The model under review builds one solid part; all positions refer to its coordinate system, in mm. A direction names the side the tool comes from. Coordinates: 2 decimals unless noted, no trailing zeros. Order: outer loops, then holes, each group sorted by start corner. A loop starts at its lowest first (then second) coordinate and runs counter-clockwise, first axis right, second up. Notation, with made-up numbers: (88, 68) - (109, 68) arc R22 ccw to (109, 91) - close; hole circle Ø7 at (18, 53). An arc over 180 degrees is marked (long way). Answer in a Markdown table with one row per item.
Autodesk Inventor part; units mm, degrees
ref_plane "YZ Plane" through (0, 0, 0) normal (1, 0, 0) x (0, 1, 0)
ref_plane "XZ Plane" through (0, 0, 0) normal (0, 1, 0) x (-1, 0, 0)
ref_plane "XY Plane" through (0, 0, 0) normal (0, 0, 1) x (1, 0, 0)
sketch "Sketch1" plane through (0, 0, 0) normal (0, 1, 0) x (-1, 0, 0)
  line L0 (-41.5, -207.85) -> (-41.5, -204.85)
  line L1 (-44.5, -201.85) -> (-51.2, -201.85)
  line L2 (-54.2, -204.85) -> (-54.2, -207.85)
  line L3 (-57.2, -210.85) -> (-61.5, -210.85)
  arc A0 (-41.5, -207.85) -> (-38.5, -210.85) centre (-38.5, -207.85) ccw
  arc A1 (-41.5, -204.85) -> (-44.5, -201.85) centre (-44.5, -204.85) ccw
  arc A2 (-51.2, -201.85) -> (-54.2, -204.85) centre (-51.2, -204.85) ccw
  arc A3 (-57.2, -210.85) -> (-54.2, -207.85) centre (-57.2, -207.85) ccw
  line L4 (41.5, -207.85) -> (41.5, -204.85)
  line L5 (44.5, -201.85) -> (51.2, -201.85)
  line L6 (54.2, -204.85) -> (54.2, -207.85)
  line L7 (61.5, -210.85) -> (57.2, -210.85)
  line L8 (38.5, -210.85) -> (-38.5, -210.85)
  arc A4 (54.2, -207.85) -> (57.2, -210.85) centre (57.2, -207.85) ccw
  arc A5 (54.2, -204.85) -> (51.2, -201.85) centre (51.2, -204.85) ccw
  arc A6 (44.5, -201.85) -> (41.5, -204.85) centre (44.5, -204.85) ccw
  arc A7 (38.5, -210.85) -> (41.5, -207.85) centre (38.5, -207.85) ccw
  line L9 (44.75, 48.15) -> (25.05, 48.15)
  line L10 (25.05, 48.15) -> (25.05, 57.15)
  line L11 (25.05, 57.15) -> (44.75, 57.15)
  line L12 (44.75, 57.15) -> (44.75, 48.15)
  line L13 (-25.05, 48.15) -> (-44.75, 48.15)
  line L14 (-44.75, 48.15) -> (-44.75, 57.15)
  line L15 (-44.75, 57.15) -> (-25.05, 57.15)
  line L16 (-25.05, 57.15) -> (-25.05, 48.15)
  line L17 (44.75, 48.15) -> (63, 48.15)
  line L18 (25.05, 48.15) -> (-25.05, 48.15)
  line L19 (-44.75, 48.15) -> (-63, 48.15)
  line L20 (63, -209.35) -> (63, 48.15)
  line L21 (-63, -209.35) -> (-63, 48.15)
  arc A8 (61.5, -210.85) -> (63, -209.35) centre (61.5, -209.35) ccw
  arc A9 (-63, -209.35) -> (-61.5, -210.85) centre (-61.5, -209.35) ccw
  point P0 (0, 0)
  point P1 (-47.85, -207.15)
  point P2 (47.85, -207.85)
  point P3 (34.9, 57.15)
  point P4 (-34.9, 57.15)
  point P5 (-59.35, -210.85)
  point P6 (0, -210.85)
  point P7 (59.35, -210.85)
  point P8 (0, 48.15)
  point P9 (-47.85, -201.85)
  point P10 (47.85, -201.85)
  dimension "d3" = 12.7
  dimension "d5" = 3
  dimension "d7" = 12.7
  dimension "d9" = 3
  dimension "d10" = 9
  dimension "d11" = 19.7
  dimension "d13" = 9
  dimension "d14" = 19.7
  dimension "d16" = 1.5
  dimension "d17" = 126
  dimension "d20" = 18.25
  dimension "d21" = 18.25
  dimension "d22" = 57.15
  dimension "d23" = 9
  dimension "d24" = 9
  dimension "d27" = 250
  dimension "d28" = 250
  dimension "d53" = 83
  dimension "d54" = 3.7
extrude "base" add sketch "Sketch1" along normal blind 5
sketch "Sketch2" plane through (0, 5, 0) normal (0, 1, 0) x (1, 0, 0)
  circle A0 centre (0, -26.65) radius 9
  line L0 (-25.05, -48.15) -> (25.05, -48.15)
  line L1 (0, -26.65) -> (-33, -26.65) construction
  point P0 (0, 0)
  dimension "d31" = 18
  dimension "d32" = 21.5
  dimension "d52" = 33
extrude "Poke Hole" cut sketch "Sketch2" against normal up to surface (5 mm away)
pattern_linear "Rectangular Pattern1" count 2 spacing 33 along (0, 0, -1) of "Poke Hole"
sketch "Sketch3" plane through (0, 5, 0) normal (0, 1, 0) x (1, 0, 0)
  circle A0 centre (0, 17.45) radius 1.5
  circle A1 centre (0, 6.35) radius 9
  circle A2 centre (-9.6129, 0.8) radius 1.5
  circle A3 centre (9.6129, 0.8) radius 1.5
  point P0 (0, 0)
  point P1 (0, 6.35)
  dimension "d41" = 3
  dimension "d42" = 11.1
  dimension "d45" = 360
extrude "Mount Holes" cut sketch "Sketch3" against normal up to surface (5 mm away) contours A0 | A2 | A3
pattern_linear "Rectangular Pattern2" count 2 spacing 33 along (0, 0, 1) of "Mount Holes"
sketch "Sketch4" plane through (0, 5, 0) normal (0, 1, 0) x (1, 0, 0)
  circle A0 centre (-44.775, -21.6952) radius 1.65
  circle A1 centre (-25.025, -21.6952) radius 1.65
  line L0 (-44.775, -21.6952) -> (-25.025, -21.6952) construction
  circle A2 centre (0, 17.45) radius 1.5 construction
  circle A3 centre (-34.9, 21.6952) radius 1.65
  line L1 (-63, 209.35) -> (-63, -48.15)
  line L2 (-25.05, -48.15) -> (25.05, -48.15) construction
  line L3 (-44.75, -48.15) -> (-25.05, -48.15) construction
  line L4 (-44.775, -21.6952) -> (-25.025, -21.6952) construction
  line L5 (-34.9, 21.6952) -> (-34.9, -21.6952) construction
  point P0 (0, 0)
  point P1 (-34.9, -48.15)
  point P2 (-34.9, 0)
  dimension "d55" = 3.3
  dimension "d56" = 3.3
  dimension "d57" = 19.75
  dimension "d58" = 3.3
  dimension "d59" = 44.5
extrude "PCB mount holes" cut sketch "Sketch4" against normal up to surface (5 mm away)
pattern_linear "Rectangular Pattern3" count 2 spacing 66 along (1, 0, 0) of "PCB mount holes"
equation "\"d7\" = d3"
equation "\"d9\" = d5"
equation "\"d10\" = d23"
equation "\"d13\" = d23"
equation "\"d14\" = d11"
equation "\"d21\" = d20"
equation "\"d24\" = d23"
equation "\"d37\" = d52"
equation "\"d40\" = d52"
equation "\"d51\" = d52"
equation "\"d56\" = d55"
equation "\"d58\" = d55"
equation "\"d66\" = 2 * d52"
properties part number "front_wall_2poke" material "PPS Plastic"
Item 1: Mouldability with a two-part tool opening along X and no side actions: class faces 6 (the face through (-63, 2, -82)), 7 (the face through (54, 2, 48.15)), 8 (the face through (-25.05, 2, 53)), 9 (the face through (63, 2, -82)) as +X half, -X half, draft (parallel to the pull), parting line (faces both ways), or undercut.
Check values:
| item | result |
|---|---|
| face 6 | -X half |
| face 7 | draft |
| face 8 | undercut |
| face 9 | +X half |
Item 2: We need section A-A, the plane x = -18. Write out the cut boundary in (y, z), then the cut area to 4 significant figures.
Check values:
| item | result |
|---|---|
| outline | (0, -210.85) - (5, -210.85) - (5, 48.15) - (0, 48.15) - close |
| area | 1,295 mm^2 |
Item 3: Clearance check with flat-ended pins moving along their axes: pin 1 Ø3 at (x, y) = (46.5, 1) entering from -Z; pin 2 Ø1.5 at (x, y) = (-11.5, 2.5) entering from +Z. State where each tip first meets the part, or that it passes through.
Check values:
| item | result |
|---|---|
| pin 1 | z = -201.85 |
| pin 2 | z = 48.15 |
Item 4: Tool access review of faces 1 (the face through (0, 2, 48.15)), 2 (the face through (-48, 2, -201.85)), 3 (the face through (-44.75, 2, 53)), 4 (the face through (44.75, 2, 53)), 5 (the face through (-1.172, 2.535, 17.727)): name each direction out of +Z, -Z, +X, -X, +Y, -Y from which nothing blocks a thin tool from reaching the whole face with its end or side.
Check values:
| item | result |
|---|---|
| face 1 | +Z, +Y, -Y |
| face 2 | -Z, +Y, -Y |
| face 3 | +Z, -X, +Y, -Y |
| face 4 | +Z, +X, +Y, -Y |
| face 5 | +Y, -Y |
Item 5: To check wall thickness, follow line 1 (X direction, y = 3.45, z = 26.65); line 2 (X direction, y = 1.95, z = 32.2); line 3 (Z direction, x = 23, y = 4.25). State the ranges of each line that lie inside material, in increasing order. Write a range as from..to.
Check values:
| item | result |
|---|---|
| line 1 | -63..-9, 9..63 |
| line 2 | -63..-11.11, -8.11..-7.09, 7.09..8.11, 11.11..63 |
| line 3 | -210.85..48.15 |
Item 6: We need section B-B, the plane y = 3.6. State how many separate pieces and enclosed holes the cut face has, then the cut area to 3 significant figures.
Check values:
| item | result |
|---|---|
| separate pieces | 1 |
| enclosed holes | 14 |
| area | 32,200 mm^2 |
